Geometry: final body of the model. Coordinates: model frame, mm. Face numbers are marked on the shaded views. Round coordinates to 2 decimals unless told otherwise and drop trailing zeros. Loops run counter-clockwise (first coordinate to the right, second up) from the corner with the lowest first, then second, coordinate; pieces in that order, holes last. Notation, with made-up numbers: M 83.5,-37 L 120.5,-37 A7 ccw 120.5,-33 Z; hole C 77,45.5 d3. An arc over 180 degrees is marked long. Return JSON: item names as keys, results as strings.
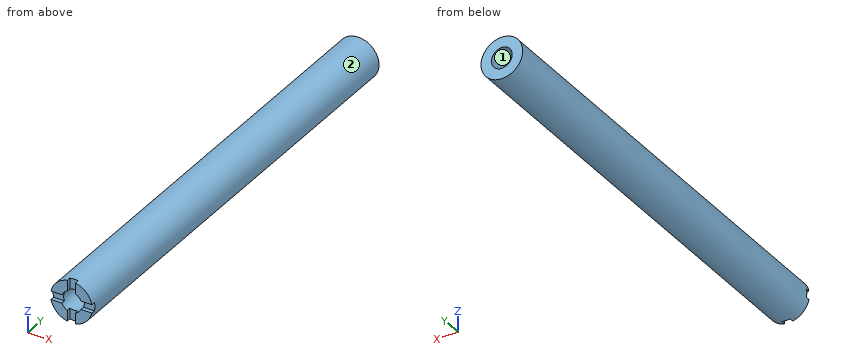
from build123d import *

# Parameters (mm, degrees)
F0_R     = 12.7
F0_R_2   = 6.35
F1_DEPTH = 279.4
F3_DEPTH = 2.54


with BuildPart() as f1:
    # F0 (on Front) → F1 (new body)
    with BuildSketch(Plane.XZ):
        Circle(F0_R)
        Circle(F0_R_2, mode=Mode.SUBTRACT)
    extrude(amount=F1_DEPTH)

    # F2 (on face) → F3 (cut)
    with BuildSketch(Plane.XZ.offset(279.4)):
        with BuildLine():
            Line((2.54, 5.8198711326), (2.54, 12.4434078933))
            ThreePointArc((2.54, 12.4434078933), (0, 12.7), (-2.54, 12.4434078933))
            Line((-2.54, 12.4434078933), (-2.54, 5.8198711326))
            ThreePointArc((-2.54, 5.8198711326), (0, 6.35), (2.54, 5.8198711326))
        make_face()
        with BuildLine():
            Line((-5.8198711326, 2.54), (-12.4434078933, 2.54))
            ThreePointArc((-12.4434078933, 2.54), (-12.7, 0), (-12.4434078933, -2.54))
            Line((-12.4434078933, -2.54), (-5.8198711326, -2.54))
            ThreePointArc((-5.8198711326, -2.54), (-6.35, 0), (-5.8198711326, 2.54))
        make_face()
        with BuildLine():
            ThreePointArc((-2.54, -12.4434078933), (0, -12.7), (2.54, -12.4434078933))
            Line((2.54, -12.4434078933), (2.54, -5.8198711326))
            ThreePointArc((2.54, -5.8198711326), (0, -6.35), (-2.54, -5.8198711326))
            Line((-2.54, -5.8198711326), (-2.54, -12.4434078933))
        make_face()
        with BuildLine():
            ThreePointArc((12.4434078933, -2.54), (12.6356891432, -1.2764638175), (12.7, 0))
            ThreePointArc((12.7, 0), (12.6356891432, 1.2764638175), (12.4434078933, 2.54))
            Line((12.4434078933, 2.54), (5.8198711326, 2.54))
            ThreePointArc((5.8198711326, 2.54), (6.2160550871, 1.2973662374), (6.35, 0))
            ThreePointArc((6.35, 0), (6.2160550871, -1.2973662374), (5.8198711326, -2.54))
            Line((5.8198711326, -2.54), (12.4434078933, -2.54))
        make_face()
    extrude(amount=-F3_DEPTH, mode=Mode.SUBTRACT)


solid = f1.part
Q1. Section query B-B (x = 0). Output: boundary loops of the cut face in (y, z).
Determined:
{"outline": "M -276.86,-12.7 L 0,-12.7 L 0,-6.35 L -276.86,-6.35 Z; M -276.86,6.35 L 0,6.35 L 0,12.7 L -276.86,12.7 Z"}
Q2. Section query C-C (y = -257). Output: boundary loops of the cut face in (x, z), plus the area to 3 significant figures.
Determined:
{"outline": "C 0,0 d25.4; hole C 0,0 d12.7", "area": "380 mm^2"}
Q3. Section query A-A (z = 0). Output: boundary loops of the cut face in (x, y).
Determined:
{"outline": "M -12.7,-276.86 L -6.35,-276.86 L -6.35,0 L -12.7,0 Z; M 6.35,-276.86 L 12.7,-276.86 L 12.7,0 L 6.35,0 Z"}
Q4. Pull-direction query (X, two-part tool) for the marked faces 1 and 2; classes: pulls with the +X half, pulls with the -X half, needs draft (parallel to the pull), parting line crosses it, or undercut.
Determined:
{"face 1": "undercut", "face 2": "parting line crosses it"}
Q5. Material intervals for L1, parallel to X at y = -233.5, z = -0.75; L2, parallel to Z at x = 0, y = -200.5; L3, parallel to Z at x = -2.75, y = -237.5, sorted ascending.
Determined:
{"L1": "x = -12.68 to -6.31, 6.31 to 12.68", "L2": "z = -12.7 to -6.35, 6.35 to 12.7", "L3": "z = -12.4 to -5.72, 5.72 to 12.4"}
Q6. Pin query (flat end, axial travel): pin 1 (0.8 mm diameter, centred on x = 10, y = -278, fed in from +Z); pin 2 (3 mm diameter, centred on y = -278.5, z = 10.5, fed in from +X); pin 3 (3 mm diameter, centred on y = -278, z = -9, fed in from -X); pin 4 (7.5 mm diameter, centred on x = 0, z = 0, fed in from -Y). Return the tip coordinate at first contact, or that it passes through.
Determined:
{"pin 1": "stops at z = 8.31", "pin 2": "stops at x = 8.96", "pin 3": "stops at x = -10.25", "pin 4": "passes through"}
